Check sheet for the modelled part. Datum: model origin and axes. Units: mm. A direction names the side the tool comes from. Round coordinates to 2 decimals unless told otherwise and drop trailing zeros. Loops run counter-clockwise (first coordinate to the right, second up) from the corner with the lowest first, then second, coordinate; pieces in that order, holes last. Notation, with made-up numbers: M 69,15 L 74,15 A10 cw 74,30 Z; hole C 70,-1 d4. An arc over 180 degrees is marked long. Write item = value, one per line. Start each with the question number.
(1) Go/stop test with flat-tipped pins: P1, Ø8, axis at x = -68, z = 19, coming from the +Y side; P2, Ø12, axis at x = 5, y = 19, coming from the -Z side; P3, Ø2, axis at x = -100, z = -7.5, coming from the +Y side. Record where each tip stops, or that it passes through.
(2) Cross-section at A-A on x = -143.5. Record the boundary of the cut face in (y, z), plus the area to 3 significant figures.
(3) Scan lines: L1, parallel to Y at x = 20.5, z = 3; L2, parallel to Y at x = 123.5, z = -1; L3, parallel to X at y = -23, z = 16. Record each from-to range of solid material in increasing order. Write a range as from..to.
(4) Set-up check for faces 1 (the face through (82.01, 11.72, 22.29)), 2 (the face through (-82, 24, -8)), 3 (the face through (165, 0, 0)): record each of +Z, -Z, +X, -X, +Y, -Y from which the full face is reachable in a straight line by a thin tool's end or side.
from build123d import *

# Parameters (mm, degrees)
SKETCH1_W = 330
SKETCH1_H = 25


with BuildPart() as part:
    # Sketch1 → Revolve1 (revolve)
    with BuildSketch(Plane.XY, mode=Mode.PRIVATE) as revolve1_sk:
        with Locations((0, 12.5)):
            Rectangle(SKETCH1_W, SKETCH1_H)
    revolve(revolve1_sk.sketch.rotate(Axis((-165, 0, 0), (1, 0, 0)), 90), axis=Axis((-165, 0, 0), (1, 0, 0)))

    # Sketch2 → Revolve2 (revolve)
    with BuildSketch(Plane.XY):
        Polygon((-82, 0), (-82, 30.119743804), (82, 30.119743804), (82, 0.119743804), align=None)
    revolve(axis=Axis((82, 0.119743804, 0), (-0.9999997334441394, -0.0007301449514384814, 0)))


solid = part.part
Result:
q1.P1 = 26.12
q1.P2 = -27.13
q1.P3 = 24.14
q2.outline = C 0,0 d50
q2.area = 1,960 mm^2
q3.L1 = -29.82..29.97
q3.L2 = -24.98..24.98
q3.L3 = -81.96..82.04
q4.face_1 = +X
q4.face_2 = -X
q4.face_3 = +Z, -Z, +X, +Y, -Y
